Check sheet for the modelled part. Datum: model origin and axes. Units: mm. A direction names the side the tool comes from. Give positions to 0.01 mm unless a question says otherwise; leave off trailing zeros. Order: outer loops, then holes, each group sorted by start corner. A loop starts at its lowest first (then second) coordinate and runs counter-clockwise, first axis right, second up.
```python
from build123d import *

# Parameters (mm, degrees)
SKETCH2_W             = 39.3827
SKETCH2_H             = 7.62
BOSS_EXTRUDE2_DEPTH   = 4.064
BOSS_EXTRUDE2_2_DEPTH = 4.064
BOSS_EXTRUDE3_DEPTH   = 2.54
BOSS_EXTRUDE4_DEPTH   = 33.02
SKETCH4_W             = 12.7
SKETCH4_H             = 2.54
CUT_EXTRUDE2_DEPTH    = 17.78
CUT_EXTRUDE3_REACH    = 74.621
SKETCH5_R             = 2.54
SKETCH5_R_2           = 1.143


with BuildPart() as part:
    # Sketch2 → Boss-Extrude2 (new body)
    with BuildSketch(Plane(origin=(0, 0, 0), x_dir=(1, 0, 0), z_dir=(0, 1, 0))):
        with Locations((19.69135, 3.81)):
            Rectangle(SKETCH2_W, SKETCH2_H)
    extrude(amount=BOSS_EXTRUDE2_DEPTH)



with BuildPart() as body_2:
    # Sketch2 → Boss-Extrude2 2 (new body)
    with BuildSketch(Plane(origin=(0, 0, 0), x_dir=(1, 0, 0), z_dir=(0, 1, 0))):
        with Locations((19.69135, 72.39)):
            Rectangle(SKETCH2_W, SKETCH2_H)
    extrude(amount=BOSS_EXTRUDE2_2_DEPTH)


with BuildPart() as part_1:
    add(part.part)

    add(body_2.part)  # Boss-Extrude3 merges body 2
    # Sketch2<3> → Boss-Extrude3 (add)
    with BuildSketch(Plane(origin=(0, 0, 0), x_dir=(1, 0, 0), z_dir=(0, 1, 0))):
        with BuildLine():
            Line((0, 34.29), (0, 7.62))
            Line((0, 7.62), (39.3827, 7.62))
            Line((39.3827, 7.62), (39.3827, 68.58))
            Line((39.3827, 68.58), (0, 68.58))
            Line((0, 68.58), (0, 41.91))
            ThreePointArc((0, 41.91), (3.81, 38.1), (0, 34.29))
        make_face()
    extrude(amount=BOSS_EXTRUDE3_DEPTH)

    # Sketch2<8> → Boss-Extrude4 (add)
    with BuildSketch(Plane(origin=(0, 0, 0), x_dir=(1, 0, 0), z_dir=(0, 1, 0))):
        Polygon((6.107856951, 51.308), (6.107856951, 38.1), (6.107856951, 24.892), (23.265414456, 24.892), (23.265414456, 51.308), align=None)
        Polygon((8.533414456, 30.48), (8.533414456, 38.1), (8.533414456, 45.72), (21.233414456, 45.72), (21.233414456, 30.48), align=None, mode=Mode.SUBTRACT)
    extrude(amount=BOSS_EXTRUDE4_DEPTH)

    # Sketch4 → Cut-Extrude2 (cut)
    with BuildSketch(Plane(origin=(0, 2.54, 0), x_dir=(1, 0, 0), z_dir=(0, 1, 0))):
        with Locations((14.883414456, 46.99)):
            Rectangle(SKETCH4_W, SKETCH4_H)
        with Locations((14.883414456, 29.21)):
            Rectangle(SKETCH4_W, SKETCH4_H)
    extrude(amount=CUT_EXTRUDE2_DEPTH, mode=Mode.SUBTRACT)

    # Cut-Extrude3: up to this face of the body (flat: up to its plane)
    cut_extrude3_end = Plane(part_1.part.faces().sort_by_distance((14.686635703, 17.78, -24.892))[0])
    # Sketch5 → Cut-Extrude3 (cut, up to the picked face)
    with BuildSketch(Plane(origin=(0, 0, -51.308), x_dir=(-1, 0, 0), z_dir=(0, 0, -1)), mode=Mode.PRIVATE) as cut_extrude3_sk1:
        with Locations((-14.686635703, 29.718)):
            Circle(SKETCH5_R)
    cut_extrude3_tool1 = split(extrude(cut_extrude3_sk1.sketch, amount=-CUT_EXTRUDE3_REACH, mode=Mode.PRIVATE), bisect_by=cut_extrude3_end, keep=Keep.BOTH, mode=Mode.PRIVATE)
    # Sketch5 → Cut-Extrude3 (cut, up to the picked face)
    with BuildSketch(Plane(origin=(0, 0, -51.308), x_dir=(-1, 0, 0), z_dir=(0, 0, -1)), mode=Mode.PRIVATE) as cut_extrude3_sk2:
        with Locations((-14.686635703, 24.257)):
            Circle(SKETCH5_R_2)
    cut_extrude3_tool2 = split(extrude(cut_extrude3_sk2.sketch, amount=-CUT_EXTRUDE3_REACH, mode=Mode.PRIVATE), bisect_by=cut_extrude3_end, keep=Keep.BOTH, mode=Mode.PRIVATE)
    add(cut_extrude3_tool1.solids().sort_by(Axis((14.686636, 29.718, -51.308), (0, 0, 1)))[0], mode=Mode.SUBTRACT)
    add(cut_extrude3_tool2.solids().sort_by(Axis((14.686636, 24.257, -51.308), (0, 0, 1)))[0], mode=Mode.SUBTRACT)


solid = part_1.part
```
(1) Set-up check for faces 1 (the face through (19, 4.064, -4)), 2 (the face through (15, 27, -45.72)), 3 (the face through (19, 3, -7.62)): record each of +Z, -Z, +X, -X, +Y, -Y from which the full face is reachable in a straight line by a thin tool's end or side.
Response values:
face 1: +Z, +X, -X, +Y
face 2: +Y
face 3: +X, -X, +Y
(2) Cross-section at D-D on y = 28. Enter the section's corners in (x, z).
Response values:
outline: (6.11, -51.31) - (12.82, -51.31) - (12.82, -45.72) - (8.53, -45.72) - (8.53, -30.48) - (12.82, -30.48) - (12.82, -24.89) - (6.11, -24.89) - close; (16.56, -51.31) - (23.27, -51.31) - (23.27, -24.89) - (16.56, -24.89) - (16.56, -30.48) - (21.23, -30.48) - (21.23, -45.72) - (16.56, -45.72) - close
(3) Cross-section at C-C on x = 32. Enter the section's corners in (y, z), then the cut area to 3 significant figures.
Response values:
outline: (0, -76.2) - (4.06, -76.2) - (4.06, -68.58) - (2.54, -68.58) - (2.54, -7.62) - (4.06, -7.62) - (4.06, 0) - (0, 0) - close
area: 217 mm2
(4) Gauge pin test, flat ends, axial feed: pin 1 Ø1.5 at (x, z) = (19.5, -42.5) entering from +Y; pin 2 Ø10 at (x, y) = (13, 25) entering from +Z; pin 3 Ø8 at (x, y) = (14.69, 29.72) entering from -Z. Record the tip position at first contact, or that the pin passes through.
Response values:
pin 1: stops at y = 2.54
pin 2: stops at z = -24.89
pin 3: stops at z = -51.31
(5) Cross-section at B-B on y = 9. Enter the section's corners in (x, z), then the cut area to 3 significant figures.
Response values:
outline: (6.11, -51.31) - (23.27, -51.31) - (23.27, -24.89) - (6.11, -24.89) - close; hole (8.53, -48.26) - (21.23, -48.26) - (21.23, -27.94) - (8.53, -27.94) - close
area: 195 mm2
(6) Release check for a two-part mould opening along X. For faces 4 (the face through (0, 2, -17)), 5 (the face through (14.93, 23.14, -48.55)), 6 (the face through (15, 18, -51.308)) record: released by +X, released by -X, zero draft, split by the parting line, or undercut.
Response values:
face 4: released by -X
face 5: undercut
face 6: zero draft
(7) Material ranges on L1, parallel to Z at x = 9, y = 28; L2, parallel to Z at x = 14, y = 16.5; L3, parallel to X at y = 4, z = -34, recorded low to high.
Response values:
L1: z = -51.31 to -45.72, -30.48 to -24.89
L2: z = -51.31 to -48.26, -27.94 to -24.89
L3: x = 6.11 to 8.53, 21.23 to 23.27
(8) Cross-section at A-A on z = -38.1. Enter the section's corners in (x, y).
Response values:
outline: (3.81, 0) - (39.38, 0) - (39.38, 2.54) - (23.27, 2.54) - (23.27, 33.02) - (21.23, 33.02) - (21.23, 2.54) - (8.53, 2.54) - (8.53, 33.02) - (6.11, 33.02) - (6.11, 2.54) - (3.81, 2.54) - close
